```python
from build123d import *

# Parameters (mm, degrees)
SKETCH_R        = 17.5
PAD_DEPTH       = 20
SKETCH001_R     = 32
POCKET_DEPTH    = 18.5
SKETCH002_R     = 0.75
SKETCH002_W     = 22.6
SKETCH002_H     = 12.2
POCKET001_DEPTH = 5
SKETCH005_R     = 17.5
PAD001_DEPTH    = 18
SKETCH006_R     = 16.3
POCKET002_DEPTH = 18


with BuildPart() as part:
    # Sketch → Pad (new body)
    with BuildSketch(Plane.XY):
        Circle(SKETCH_R)
    extrude(amount=PAD_DEPTH)

    # Sketch001 (on Face3 of Pad) → Pocket (cut)
    with BuildSketch(Plane.XY.offset(20)):
        Circle(SKETCH001_R)
    extrude(amount=-POCKET_DEPTH, mode=Mode.SUBTRACT)

    # Sketch002 (on Face2 of Pocket) → Pocket001 (cut)
    with BuildSketch(Plane(origin=(0, 0, 0), x_dir=(1, 0, 0), z_dir=(0, 0, -1))):
        with Locations((-14.4, 0)):
            Circle(SKETCH002_R)
        with Locations((14.4, 0)):
            Circle(SKETCH002_R)
        Rectangle(SKETCH002_W, SKETCH002_H)
    extrude(amount=-POCKET001_DEPTH, mode=Mode.SUBTRACT)

    # Sketch005 (on Face3 of Pocket001) → Pad001 (join)
    with BuildSketch(Plane.XY.offset(1.5)):
        Circle(SKETCH005_R)
    extrude(amount=PAD001_DEPTH)

    # Sketch006 (on Face4 of Pad001) → Pocket002 (cut)
    with BuildSketch(Plane.XY.offset(19.5)):
        Circle(SKETCH006_R)
    extrude(amount=-POCKET002_DEPTH, mode=Mode.SUBTRACT)


solid = part.part
```
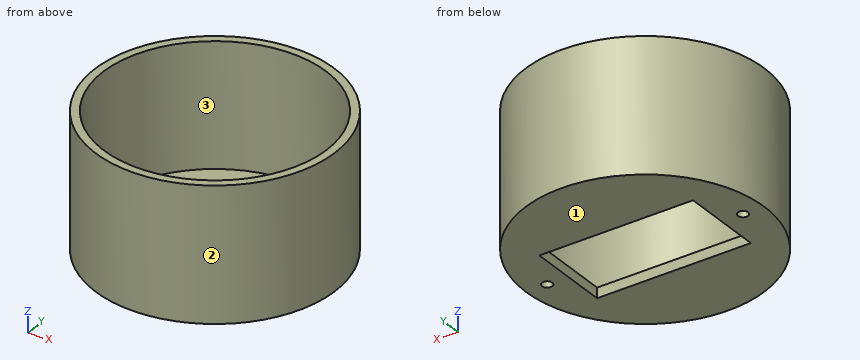
Work out the finished part from the listing and answer in its coordinate system (mm). Face numbers are marked on the shaded views. Coordinates: 2 decimals unless noted, no trailing zeros. Order: outer loops, then holes, each group sorted by start corner. A loop starts at its lowest first (then second) coordinate and runs counter-clockwise, first axis right, second up. Notation, with made-up numbers: M 76.25,71.25 L 134.25,71.25 A18 ccw 134.25,99.25 Z; hole C 47,-28.5 d6. An arc over 180 degrees is marked long. Use CSV: the item, a comma, the result in double quotes.
1) Consider line 1 (X direction, y = -0.5, z = 7.5); line 2 (Y direction, x = 0, z = 12.75); line 3 (Z direction, x = 1, y = -8). Determine where each line is inside the solid, lowest interval first. Write a range as [from, to].
Worked out:
line 1,"x = [-17.49, -16.29], [16.29, 17.49]"
line 2,"y = [-17.5, -16.3], [16.3, 17.5]"
line 3,"z = [0, 1.5]"
2) Section B-B on y = 0 is taken. Write down the section's boundary in (x, z), plus the area to 3 significant figures.
Worked out:
outline,"M -17.5,0 L -15.15,0 L -15.15,1.5 L -16.3,1.5 L -16.3,19.5 L -17.5,19.5 Z; M -13.65,0 L -11.3,0 L -11.3,1.5 L -13.65,1.5 Z; M 11.3,0 L 13.65,0 L 13.65,1.5 L 11.3,1.5 Z; M 15.15,0 L 17.5,0 L 17.5,19.5 L 16.3,19.5 L 16.3,1.5 L 15.15,1.5 Z"
area,"57.3 mm^2"
3) Flat-ended cylindrical pins translate along their axes: pin 1 Ø10 at (x, z) = (-7, 2.5) entering from -Y; pin 2 Ø2 at (y, z) = (-5, 13) entering from -X; pin 3 Ø1.2 at (x, z) = (2.5, 0.5) entering from +Y. Find the tip coordinate at first contact, or state that the pin passes through.
Worked out:
pin 1,"stops at y = -17.39"
pin 2,"stops at x = -17.04"
pin 3,"stops at y = 17.4"
4) Section D-D on y = 8.5 is taken. Write down the section's boundary in (x, z), plus the area to 3 significant figures.
Worked out:
outline,"M -15.3,0 L 15.3,0 L 15.3,19.5 L 13.91,19.5 L 13.91,1.5 L -13.91,1.5 L -13.91,19.5 L -15.3,19.5 Z"
area,"95.9 mm^2"
5) Section A-A on x = 0 is taken. Write down the section's boundary in (y, z).
Worked out:
outline,"M -17.5,0 L -6.1,0 L -6.1,1.5 L -16.3,1.5 L -16.3,19.5 L -17.5,19.5 Z; M 6.1,0 L 17.5,0 L 17.5,19.5 L 16.3,19.5 L 16.3,1.5 L 6.1,1.5 Z"
6) Section C-C on z = 8.75 is taken. Write down the section's boundary in (x, y).
Worked out:
outline,"C 0,0 d35; hole C 0,0 d32.6"
7) Determine the mould class of the marked faces 1, 2 and 3 for opening direction Y: released by +Y, released by -Y, zero draft, split by the parting line, or undercut.
Worked out:
face 1,"zero draft"
face 2,"split by the parting line"
face 3,"undercut"
